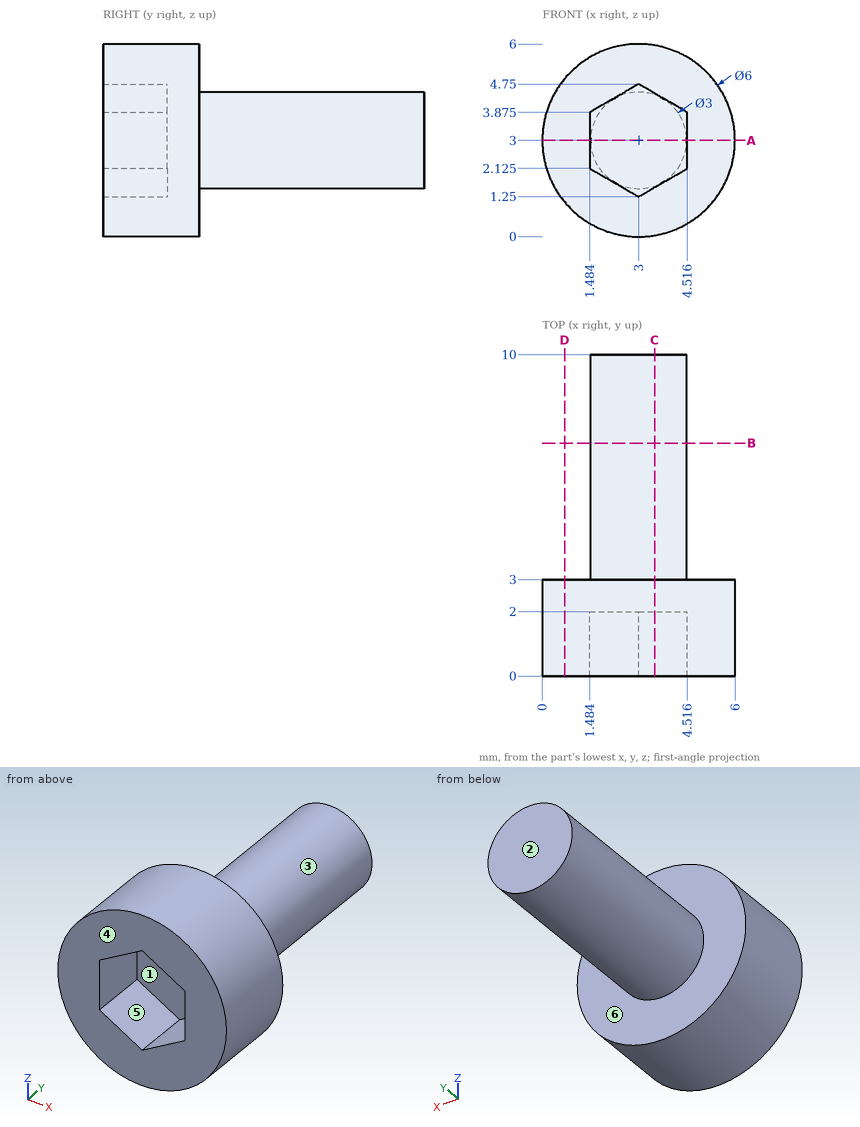
Can you work these out from the drawing? Everything is in mm from the part's minimum corner. A direction names the side the tool comes from. Round coordinates to 2 decimals unless told otherwise and drop trailing zeros. Loops run counter-clockwise (first coordinate to the right, second up) from the corner with the lowest first, then second, coordinate; pieces in that order, holes last. Notation, with made-up numbers: (4.5, -40) -> (23.5, -40) arc R11 cw to (23.5, -33) -> close; hole circle Ø4 at (89.25, 51.25). An arc over 180 degrees is marked (long way). Use CSV: the item, a comma, the result in double quotes.
(1) For the marked faces 4, 5 and 6, which set-ups out of +Z, -Z, +X, -X, +Y, -Y let a thin tool reach every point of the face, with its end or its side?
Return value:
face 4,"+Z, -Z, +X, -X, -Y"
face 5,"-Y"
face 6,"+Y"
(2) Suppose I cut it at A-A on z = 3. Write out the boundary of the cut face in (x, y) (1 decimal).
Return value:
outline,"(0, 0) -> (1.5, 0) -> (1.5, 2) -> (4.5, 2) -> (4.5, 0) -> (6, 0) -> (6, 3) -> (4.5, 3) -> (4.5, 10) -> (1.5, 10) -> (1.5, 3) -> (0, 3) -> close"
(3) Suppose I cut it at D-D on x = 0.7. Write out the boundary of the cut face in (y, z).
Return value:
outline,"(0, 1.07) -> (3, 1.07) -> (3, 4.93) -> (0, 4.93) -> close"
(4) If I drill on probe 1 along Y at (x, z) = (1.3, 4.8); probe 2 along X at (y, z) = (1.75, 3.4) (1 decimal); probe 3 along Y at (x, z) = (3.95, 3.55), over which ranges is the centre line in solid material (lowest first)? Write a range as [from, to].
Return value:
probe 1,"y = [0, 3]"
probe 2,"x = [0, 1.5], [4.5, 6]"
probe 3,"y = [2, 10]"
(5) Suppose I cut it at C-C on x = 3.5. Write out the boundary of the cut face in (y, z) (1 decimal).
Return value:
outline,"(0, 0) -> (3, 0) -> (3, 1.6) -> (10, 1.6) -> (10, 4.4) -> (3, 4.4) -> (3, 6) -> (0, 6) -> (0, 4.5) -> (2, 4.5) -> (2, 1.5) -> (0, 1.5) -> close"
(6) Will these pins go through, and if not, where does the flat tip stop? pin 1 Ø0.9 at (x, z) = (3, 3) entering from -Y; pin 2 Ø1 at (x, z) = (2.5, 1) entering from +Y.
Return value:
pin 1,"stops at y = 2"
pin 2,"stops at y = 3"
(7) Suppose I cut it at B-B on y = 7.25. Write out the boundary of the cut face in (x, z).
Return value:
outline,"circle Ø3 at (3, 3)"
(8) If we mould it in two halves opening along Z, with no side actions, what happens to the marked faces 1, 2 and 3? For each: +Z half, -Z half, draft (parallel to the pull), parting line (faces both ways), or undercut.
Return value:
face 1,"undercut"
face 2,"draft"
face 3,"parting line"
